Verification items for the finished model (mm, model axes). Give positions to 0.01 mm unless a question says otherwise; leave off trailing zeros. Write each loop counter-clockwise with the first axis right and the second up, starting at its lowest first coordinate (ties: lowest second). Pieces come first, ordered by that corner, then holes.
from build123d import *

# Parameters (mm, degrees)
BOSS_EXTRUDE1_DEPTH = 114.3
BOSS_EXTRUDE2_DEPTH = 76.2


with BuildPart() as part:
    # Sketch1 → Boss-Extrude1 (new body)
    with BuildSketch(Plane(origin=(0, 0, 0), x_dir=(1, 0, 0), z_dir=(0, 1, 0))):
        Polygon((-1.218394187, 0.358351231), (1.218394187, -0.358351231), (-27.449704331, -97.829886191), (-29.886492705, -97.113183728), align=None)
    extrude(amount=-BOSS_EXTRUDE1_DEPTH)

    # Sketch2 → Boss-Extrude2 (add)
    with BuildSketch(Plane(origin=(0, 0, 0), x_dir=(1, 0, 0), z_dir=(0, 1, 0))):
        Polygon((-14.584895121, -47.338197677), (-15.301597584, -49.774986051), (-14.083203397, -50.133337283), (-13.366500934, -47.696548909), align=None)
    extrude(amount=BOSS_EXTRUDE2_DEPTH)


solid = part.part
Item 1: Sectioned sample at A-A on y = 12. Record the cut outline in (x, z), then the cut area to 3 significant figures.
Answer key:
outline: (-15.3, 49.77) - (-14.58, 47.34) - (-13.37, 47.7) - (-14.08, 50.13) - close
area: 3.23 mm2
Item 2: Depth check by flat-ended pin: pin 1 (9.5 mm diameter, centred on x = -15, z = 73, fed in from +Y); pin 2 (1.5 mm diameter, centred on y = -40, z = 66, fed in from -X); pin 3 (5 mm diameter, centred on y = -67.5, z = 68.5, fed in from -X); pin 4 (4 mm diameter, centred on y = 25, z = 51.5, fed in from -X). Enter the tip coordinate at first touch or a pass-through.
Answer key:
pin 1: passes through
pin 2: stops at x = -20.96
pin 3: stops at x = -22.21
pin 4: stops at x = -15.3
Item 3: Sectioned sample at B-B on x = -3. Record the cut outline in (y, z).
Answer key:
outline: (-114.3, 5.7) - (0, 5.7) - (0, 14.7) - (-114.3, 14.7) - close
Item 4: Scan lines: line 1 along X through (y, z) = (-72, 79); line 2 along X through (y, z) = (-49, 34.5). Record each from-to range of solid material in increasing order.
Answer key:
line 1: x = -24.56 to -21.91
line 2: x = -11.47 to -8.82
